Design review of the part built by this model. Coordinates are the model's own, in mm. A direction names the side the tool comes from. Coordinates: 2 decimals unless noted, no trailing zeros. Write each loop counter-clockwise with the first axis right and the second up, starting at its lowest first coordinate (ties: lowest second). Pieces come first, ordered by that corner, then holes. Notation, with made-up numbers: (4.25, 54.25) -> (20.25, 54.25) arc R7 ccw to (20.25, 64.25) -> close; hole circle Ø1 at (8, 74.25). An arc over 180 degrees is marked (long way). One line per question, with ' | ' between items. Start each with the question number.
Q1. Add section C-C on y = -27. State the section outline as (x, z) points, and give its area (3 significant figures).
Q2. Add section A-A on z = 50.5. State the section outline as (x, y) points, and give its area (3 significant figures).
Q3. For P1, Ø5, axis at y = -80.5, z = 2.5, coming from the +X side; P2, Ø8, axis at x = -24.5, z = 18, coming from the -Y side; P3, Ø10, axis at x = 52.5, y = 77.5, coming from the +Z side, all flat-tipped, find the tip position at first contact; note any pin that passes through.
Q4. For faces 4 (the cylindrical face through (52.287, -100.035, 3.397)), 5 (the cylindrical face through (79.29, -100.04, 3.3)), 6 (the flat face through (13, -57.406, 67)), 7 (the flat face through (62.7, -130.295, 0.4)), 8 (the flat face through (52.819, -93, 4)), list the 3-axis set-ups (+Z, -Z, +X, -X, +Y, -Y) from which the entire face can be reached by the end or side of a thin tool; tool diameter is ignored.
Q5. Draft analysis for pull direction Z (two halves, no side actions). For faces 1 (the flat face through (100.171, 16, 65)), 2 (the flat face through (9, 15, 0)), 3 (the cylindrical face through (66.03, -64.1, 16.39)), state which applies: pulls with the +Z half, pulls with the -Z half, needs draft (parallel to the pull), parting line crosses it, or undercut.
Q6. Wall thickness on probe 1 along Y at (x, z) = (78, 83); probe 2 along X at (y, z) = (-11.5, 120.5); probe 3 along Y at (x, z) = (60.5, 7): over which ranges is each line inside the solid? List them lowest first.
Q7. Add section B-B on x = 13.5. State the section outline as (y, z) points.
from build123d import *

# Parameters (mm, degrees)
F0_W      = 179.383456707
F0_H      = 175.0688403845
F0_W_2    = 160.5059653521
F0_H_2    = 146.9108834863
F1_DEPTH  = 132
F3_DEPTH  = 25
F5_DEPTH  = 10
F6_DEPTH  = 10
F7_W      = 160.5059653521
F7_H      = 6.6701923497
F8_DEPTH  = 163
F9_DEPTH  = 6
F10_DEPTH = 3
F11_DEPTH = 59.8


with BuildPart() as f1:
    # F0 (on Top) → F1 (new body)
    with BuildSketch(Plane.XY):
        with Locations((10.4796737432, 16.923636198)):
            Rectangle(F0_W, F0_H)
        with Locations((12.0261907578, 19.04932037)):
            Rectangle(F0_W_2, F0_H_2, mode=Mode.SUBTRACT)
    extrude(amount=F1_DEPTH)

    # F2 (on face) → F3 (cut)
    with BuildSketch(Plane.XZ.offset(70.6107839942)):
        with BuildLine():
            Line((52.587673068, 0), (78.987672925, 0))
            ThreePointArc((78.987672925, 0), (65.7876729965, 16.3912356025), (52.587673068, 0))
        make_face()
    extrude(amount=-F3_DEPTH, mode=Mode.SUBTRACT)

    # F4 (on face) → F5 (join)
    with BuildSketch(Plane(origin=(0, 0, 0), x_dir=(1, 0, 0), z_dir=(0, 0, -1))):
        Polygon((52.587673068, 54.4061213732), (-68.2267919183, 54.4061213732), (-68.2267919183, -92.5047621131), (92.2791734338, -92.5047621131), (92.2791734338, 54.4061213732), (78.987672925, 54.4061213732), align=None)
    extrude(amount=-F5_DEPTH)

    # F6 (cut): a face of the model
    f6_faces = [f1.faces().sort_by_distance(p)[0] for p in [
        (12.0261907578, 19.04932037, 10),
    ]]
    extrude(f6_faces, amount=-F6_DEPTH, mode=Mode.SUBTRACT)

    # F7 (on face) → F8 (join)
    with BuildSketch(Plane.XZ.offset(-92.5047621131)):
        with Locations((12.0261907578, 3.3350961749)):
            Rectangle(F7_W, F7_H)
    extrude(amount=F8_DEPTH)

    # F9 (cut): a face of the model
    f9_faces = [f1.faces().sort_by_distance(p)[0] for p in [
        (12.9610636672, 17.6320948964, 6.6701923497),
    ]]
    extrude(f9_faces, amount=-F9_DEPTH, mode=Mode.SUBTRACT)

    # F10 (cut): a face of the model
    f10_faces = [f1.faces().sort_by_distance(p)[0] for p in [
        (11.1413753664, -54.4061213732, 67.3034038031),
    ]]
    extrude(f10_faces, amount=-F10_DEPTH, mode=Mode.SUBTRACT)

    # F11 (add): a face of the model
    f11_faces = [f1.faces().sort_by_distance(p)[0] for p in [
        (52.5633202811, -70.4952378869, 3.3399666354),
    ]]
    extrude(f11_faces, amount=F11_DEPTH)


solid = f1.part
Output values:
1) outline: (-79.21, 0) -> (100.17, 0) -> (100.17, 132) -> (92.28, 132) -> (92.28, 0.67) -> (-68.23, 0.67) -> (-68.23, 132) -> (-79.21, 132) -> close | area: 2,600 mm2
2) outline: (-79.21, -70.61) -> (100.17, -70.61) -> (100.17, 104.46) -> (-79.21, 104.46) -> close; hole (-68.23, -57.41) -> (92.28, -57.41) -> (92.28, 92.5) -> (-68.23, 92.5) -> close | area: 7,340 mm2
3) P1: stops at x = 79.3 | P2: stops at y = -70.61 | P3: stops at z = 0.67
4) face 4: -X, -Y | face 5: +X, -Y | face 6: +Z | face 7: +Z, -Z, +X, -X, -Y | face 8: -Y
5) face 1: needs draft | face 2: pulls with the -Z half | face 3: undercut
6) probe 1: y = -70.61 to -57.41, 92.5 to 104.46 | probe 2: x = -79.21 to -68.23, 92.28 to 100.17 | probe 3: y = 92.5 to 104.46
7) outline: (-70.61, 0) -> (104.46, 0) -> (104.46, 132) -> (92.5, 132) -> (92.5, 0.67) -> (-57.41, 0.67) -> (-57.41, 132) -> (-70.61, 132) -> close
